Read the model definition and answer for the solid it produces. Units are mm, in the model's axes. A direction names the side the tool comes from. Give positions to 0.01 mm unless a question says otherwise; leave off trailing zeros. Loops run counter-clockwise (first coordinate to the right, second up) from the corner with the lowest first, then second, coordinate; pieces in that order, holes last. Notation, with made-up numbers: (68.5, 83.25) -> (98.5, 83.25) arc R24 cw to (98.5, 93.25) -> close; hole circle Ø5 at (16.25, 24). An arc over 180 degrees is marked (long way). One line per item, written item: value. Start each with the question number.
from build123d import *

# Parameters (mm, degrees)
F2_SIZE  = 0.5
F3_R     = 0.2
F4_R     = 0.2
F5_R     = 1
F7_DEPTH = 1.5
F8_SIZE  = 1.49999


# Not quite as in the source:
# - a fillet or chamfer is up to 0.001 mm smaller than in the source, because OpenCascade refuses the exact size


with BuildPart() as f1:
    # F0 (on Top) → F1 (revolve)
    with BuildSketch(Plane.XY):
        Polygon((0, 3.5), (0, 0), (8, 0), (8, 1.75), (2, 1.75), (2, 3.5), align=None)
    revolve(axis=Axis((4, 0, 0), (-1, 0, 0)))

    # F2
    f2_edges = [f1.edges().sort_by_distance(p)[0] for p in [
        (8, -1.75, 0),
    ]]
    chamfer(f2_edges, length=F2_SIZE)

    # F3
    f3_edges = [f1.edges().sort_by_distance(p)[0] for p in [
        (2, -1.75, 0),
    ]]
    fillet(f3_edges, radius=F3_R)

    # F4
    f4_edges = [f1.edges().sort_by_distance(p)[0] for p in [
        (2, -3.5, 0),
    ]]
    fillet(f4_edges, radius=F4_R)

    # F5
    f5_edges = [f1.edges().sort_by_distance(p)[0] for p in [
        (0, -3.5, 0),
    ]]
    fillet(f5_edges, radius=F5_R)

    # F6 (on face) → F7 (cut)
    with BuildSketch(Plane(origin=(0, 0, 0), x_dir=(0, -1, 0), z_dir=(-1, 0, 0))):
        Polygon((-0.75, 2.25), (-0.75, 0.75), (-2.25, 0.75), (-2.25, -0.75), (-0.75, -0.75), (-0.75, -2.25), (0.75, -2.25), (0.75, -0.75), (2.25, -0.75), (2.25, 0.75), (0.75, 0.75), (0.75, 2.25), align=None)
    extrude(amount=-F7_DEPTH, mode=Mode.SUBTRACT)

    # F8 (size 1.5 in the source; OpenCascade refuses exactly that, so slightly less here)
    f8_edges = [f1.edges().sort_by_distance(p)[0] for p in [
        (1.5, 2.25, 0),
        (1.5, 0, 2.25),
        (1.5, 0, -2.25),
        (1.5, -2.25, 0),
    ]]
    chamfer(f8_edges, length=F8_SIZE)


solid = f1.part
Item 1: Section C-C, the plane x = 0.5 is taken. Determine the outline of the cut face in (y, z), plus the area to 3 significant figures.
Item 2: Determine the mould class of faces 4 (the cylindrical face through (1.394, 3.233, 1.341)), 5 (the flat face through (2, 0, 2.2)), 6 (the flat face through (1, -1, 0.75)) for opening direction Z: pulls with the +Z half, pulls with the -Z half, needs draft (parallel to the pull), parting line crosses it, or undercut.
Item 3: Section D-D, the plane x = 3.5 is taken. Determine the outline of the cut face in (y, z).
Item 4: For faces 1 (the cylindrical face through (4.813, 1.617, 0.67)), 2 (the flat face through (0, -1, -1)), 3 (the flat face through (1, 1, 0.75)), determine the directions among +Z, -Z, +X, -X, +Y, -Y from which every point of the face is accessible in a straight line to the end or side of a thin tool.
Item 5: Consider L1, parallel to X at y = -1.5, z = 1.5; L2, parallel to Y at x = 3.75, z = 0; L3, parallel to Z at x = 1.5, y = 3. Determine where each line is inside the solid, lowest interval first. Write a range as [from, to].
Item 6: Flat-ended cylindrical pins translate along their axes: pin 1 (1.5 mm diameter, centred on y = -2.5, z = -1, fed in from +X); pin 2 (3 mm diameter, centred on x = 3, z = -1.5, fed in from +Y); pin 3 (1.6 mm diameter, centred on x = 0.5, y = -1.5, fed in from -Z). Find the tip coordinate at first contact, or state that the pin passes through.
Computed values:
1. outline: circle Ø6.73 at (0, 0); hole (-1.75, -0.75) -> (-0.75, -0.75) -> (-0.75, -1.75) -> (0.75, -1.75) -> (0.75, -0.75) -> (1.75, -0.75) -> (1.75, 0.75) -> (0.75, 0.75) -> (0.75, 1.75) -> (-0.75, 1.75) -> (-0.75, 0.75) -> (-1.75, 0.75) -> close
1. area: 27.3 mm²
2. face 4: parting line crosses it
2. face 5: needs draft
2. face 6: undercut
3. outline: circle Ø3.5 at (0, 0)
4. face 1: +X
4. face 2: +Z, -Z, -X, +Y, -Y
4. face 3: -X
5. L1: [0, 2]
5. L2: [-1.75, 1.75]
5. L3: [-1.8, 1.8]
6. pin 1: x = 2
6. pin 2: y = 3.45
6. pin 3: z = -3.4
